For this review, take the finished solid that the model builds, in its own axes (mm). Face numbers are marked on the shaded views. A direction names the side the tool comes from. Give positions to 0.01 mm unless a question says otherwise; leave off trailing zeros. Write each loop counter-clockwise with the first axis right and the second up, starting at its lowest first coordinate (ties: lowest second). Pieces come first, ordered by that corner, then holes.
1) We need section C-C on z = 7. Give the number of separate pieces and of enclosed holes in the cut face, and give its area (3 significant figures).
2) Wall thickness on line 1 along Z through (x, y) = (-0.5, 2.25); line 2 along Z through (x, y) = (-12, -2.5); line 3 along Z through (x, y) = (-11, 0.5): over which ranges is each line inside the solid? List them lowest first.
3) Draft analysis for pull direction Z (two halves, no side actions). For the marked faces 1, 2 and 3, state which applies: pulls with the +Z half, pulls with the -Z half, needs draft (parallel to the pull), parting line crosses it, or undercut.
4) Machinability: for the marked faces 4, 5 and 6, which of the approach directions +Z, -Z, +X, -X, +Y, -Y give a long, thin tool a straight path to every point of the face, cutting with its end or side? Answer none if there is none.
5) For P1, Ø1.8, axis at x = 8.25, z = -14.29, coming from the +Y side; P2, Ø1.8, axis at x = 0, z = 18.5, coming from the -Y side; P3, Ø0.8, axis at y = 1.5, z = -20, coming from the -X side; P4, Ø1.5, axis at y = -2.5, z = -10.5, coming from the -X side, all flat-tipped, find the tip position at first contact; note any pin that passes through.
6) We need section A-A on z = 0. Give the boundary of the cut face in (x, y) (3 decimals).
7) We need section B-B on y = -3. Give the boundary of the cut face in (x, z) (3 decimals).
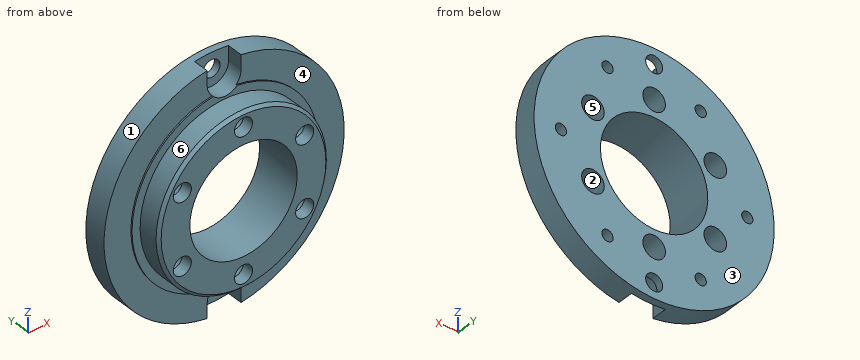
from build123d import *

# Parameters (mm, degrees)
SKETCH1_R           = 21.25
BOSS_EXTRUDE1_DEPTH = 4
SKETCH2_R           = 1.5
CUT_EXTRUDE1_DEPTH  = 4
SKETCH5_R           = 16.5
BOSS_EXTRUDE2_DEPTH = 0.25
SKETCH6_R           = 15.075
BOSS_EXTRUDE3_DEPTH = 4
CHAMFER1_SIZE       = 0.5
SKETCH7_R           = 9.5
CUT_EXTRUDE3_DEPTH  = 8.25
SKETCH8_R           = 1
CUT_EXTRUDE4_DEPTH  = 3
CIRPATTERN2_COUNT   = 6
CUT_EXTRUDE5_DEPTH  = 3
CIRPATTERN3_COUNT   = 2
SKETCH13_R          = 2
CUT_EXTRUDE6_DEPTH  = 6.25
SKETCH14_R          = 1.6
CUT_EXTRUDE7_DEPTH  = 2
CIRPATTERN4_COUNT   = 6


with BuildPart() as part:
    # Sketch1 → Boss-Extrude1 (new body)
    with BuildSketch(Plane(origin=(0, 0, 0), x_dir=(1, 0, 0), z_dir=(0, 1, 0))):
        with Locations(Location((0, 0, 0), (0, 0, 270))):
            Circle(SKETCH1_R)
    extrude(amount=BOSS_EXTRUDE1_DEPTH)

    # Sketch2 → Cut-Extrude1 (cut)
    with BuildSketch(Plane(origin=(0, 4, 0), x_dir=(1, 0, 0), z_dir=(0, 1, 0))):
        with Locations(Location((0, 18.5, 0), (0, 0, 270))):
            Circle(SKETCH2_R)
    cut_extrude1 = extrude(amount=-CUT_EXTRUDE1_DEPTH, mode=Mode.SUBTRACT)

    # Sketch5 → Boss-Extrude2 (add)
    with BuildSketch(Plane.XZ):
        with Locations(Location((0, 0, 0), (0, 0, 90))):
            Circle(SKETCH5_R)
    extrude(amount=BOSS_EXTRUDE2_DEPTH)

    # Sketch6 → Boss-Extrude3 (add)
    with BuildSketch(Plane.XZ.offset(0.25)):
        with Locations(Location((0, 0, 0), (0, 0, 270))):
            Circle(SKETCH6_R)
    extrude(amount=BOSS_EXTRUDE3_DEPTH)

    # Chamfer1
    chamfer1_edges = [part.edges().sort_by_distance(p)[0] for p in [
        (0, -4.25, 15.075),
    ]]
    chamfer(chamfer1_edges, length=CHAMFER1_SIZE)

    # Sketch7 → Cut-Extrude3 (cut)
    with BuildSketch(Plane.XZ.offset(4.25)):
        with Locations(Location((0, 0, 0), (0, 0, 270))):
            Circle(SKETCH7_R)
    extrude(amount=-CUT_EXTRUDE3_DEPTH, mode=Mode.SUBTRACT)

    # Sketch8 → Cut-Extrude4 (cut)
    with BuildSketch(Plane(origin=(0, 4, 0), x_dir=(1, 0, 0), z_dir=(0, 1, 0))):
        with Locations(Location((8.25, 14.289419162, 0), (0, 0, 270))):
            Circle(SKETCH8_R)
    cut_extrude4 = extrude(amount=-CUT_EXTRUDE4_DEPTH, mode=Mode.SUBTRACT)

    # CirPattern2: Cut-Extrude4 ×6 about axis
    cirpattern2_axis = Axis((0, 0, 0), (0, 1, 0))
    for i in range(1, CIRPATTERN2_COUNT):
        add(cut_extrude4.rotate(cirpattern2_axis, i * 360 / CIRPATTERN2_COUNT), mode=Mode.SUBTRACT)

    # Sketch11 → Cut-Extrude5 (cut)
    with BuildSketch(Plane.XZ.offset(0.25)):
        with BuildLine():
            Line((-3, -18.5), (-3, -22.883659788))
            Line((-3, -22.883659788), (3, -22.883659788))
            Line((3, -22.883659788), (3, -18.5))
            ThreePointArc((3, -18.5), (0, -15.5), (-3, -18.5))
        make_face()
    cut_extrude5 = extrude(amount=-CUT_EXTRUDE5_DEPTH, mode=Mode.SUBTRACT)

    # CirPattern3: Cut-Extrude1, Cut-Extrude5 ×2 about axis
    cirpattern3_axis = Axis((0, 0, 0), (0, 1, 0))
    add([cut_extrude1.rotate(cirpattern3_axis, i * 360 / CIRPATTERN3_COUNT) for i in range(1, CIRPATTERN3_COUNT)], mode=Mode.SUBTRACT)
    add([cut_extrude5.rotate(cirpattern3_axis, i * 360 / CIRPATTERN3_COUNT) for i in range(1, CIRPATTERN3_COUNT)], mode=Mode.SUBTRACT)

    # Sketch13 → Cut-Extrude6 (cut)
    with BuildSketch(Plane(origin=(0, 4, 0), x_dir=(1, 0, 0), z_dir=(0, 1, 0))):
        with Locations(Location((0, 12.5, 0), (0, 0, 270))):
            Circle(SKETCH13_R)
    cut_extrude6 = extrude(amount=-CUT_EXTRUDE6_DEPTH, mode=Mode.SUBTRACT)

    # Sketch14 → Cut-Extrude7 (cut)
    with BuildSketch(Plane(origin=(0, -2.25, 0), x_dir=(1, 0, 0), z_dir=(0, 1, 0))):
        with Locations(Location((0, 12.5, 0), (0, 0, 270))):
            Circle(SKETCH14_R)
    cut_extrude7 = extrude(amount=-CUT_EXTRUDE7_DEPTH, mode=Mode.SUBTRACT)

    # CirPattern4: Cut-Extrude6, Cut-Extrude7 ×6 about axis
    cirpattern4_axis = Axis((0, 0, 0), (0, 1, 0))
    add([cut_extrude6.rotate(cirpattern4_axis, i * 360 / CIRPATTERN4_COUNT) for i in range(1, CIRPATTERN4_COUNT)], mode=Mode.SUBTRACT)
    add([cut_extrude7.rotate(cirpattern4_axis, i * 360 / CIRPATTERN4_COUNT) for i in range(1, CIRPATTERN4_COUNT)], mode=Mode.SUBTRACT)


solid = part.part
Results list:
1. separate pieces: 4
1. enclosed holes: 0
1. area: 111 mm2
2. line 1: z = -15.54 to -14.44, -10.56 to -9.49, 9.49 to 10.56, 14.44 to 15.54
2. line 2: z = -9.12 to -7.34, -5.16 to 5.16, 7.34 to 9.12
2. line 3: z = -18.18 to -8.24, -4.26 to 4.26, 8.24 to 18.18
3. face 1: parting line crosses it
3. face 2: undercut
3. face 3: needs draft
4. face 4: +X, -Y
4. face 5: +Y
4. face 6: -Y
5. P1: stops at y = 1
5. P2: passes through
5. P3: stops at x = -8.21
5. P4: stops at x = -11.5
6. outline: (-21.25, 0) - (-16.5, 0) - (-16.5, -0.25) - (-15.075, -0.25) - (-15.075, -3.75) - (-14.575, -4.25) - (-9.5, -4.25) - (-9.5, 4) - (-15.5, 4) - (-15.5, 1) - (-17.5, 1) - (-17.5, 4) - (-21.25, 4) - close; (9.5, -4.25) - (14.575, -4.25) - (15.075, -3.75) - (15.075, -0.25) - (16.5, -0.25) - (16.5, 0) - (21.25, 0) - (21.25, 4) - (17.5, 4) - (17.5, 1) - (15.5, 1) - (15.5, 4) - (9.5, 4) - close
7. outline: circle Ø30.15 at (0, 0); hole circle Ø3.2 at (-10.825, -6.25); hole circle Ø3.2 at (-10.825, 6.25); hole circle Ø19 at (0, 0); hole circle Ø3.2 at (0, -12.5); hole circle Ø3.2 at (0, 12.5); hole circle Ø3.2 at (10.825, -6.25); hole circle Ø3.2 at (10.825, 6.25)
